```python
from build123d import *

# Parameters (mm, degrees)
F0_W     = 69.85
F0_H     = 95.25
F1_DEPTH = 38.1
F2_W     = 44.45
F2_H     = 73.66
F3_DEPTH = 25.4
F4_R     = 5.08
F5_R     = 4.826
F6_DEPTH = 12.7
F7_W     = 12.954
F7_H     = 6.35
F8_DEPTH = 12.7


# Not quite as in the source:
# - a feature names something its author has since deleted; it is built from what else it names


with BuildPart() as f1:
    # F0 (on Front) → F1 (new body)
    with BuildSketch(Plane.XZ):
        Rectangle(F0_W, F0_H)
    extrude(amount=F1_DEPTH)

    # F2 (on face) → F3 (cut)
    with BuildSketch(Plane(origin=(0, 0, 0), x_dir=(-1, 0, 0), z_dir=(0, 1, 0))):
        Rectangle(F2_W, F2_H)
    extrude(amount=-F3_DEPTH, mode=Mode.SUBTRACT)

    # F4
    f4_edges = [f1.edges().sort_by_distance(p)[0] for p in [
        (0, -38.1, 47.625),
        (0, 0, 47.625),
        (0, -38.1, -47.625),
        (0, 0, -47.625),
    ]]
    fillet(f4_edges, radius=F4_R)

    # F5 (on face) → F6 (cut)
    with BuildSketch(Plane.XZ.offset(38.1)):
        with Locations((-10.6567444081, 13.887990205)):
            Circle(F5_R)
        with Locations((9.5055226038, 14.3169752002)):
            Circle(F5_R)
    extrude(amount=-F6_DEPTH, mode=Mode.SUBTRACT)

    # F7 (on face) → F8 (cut)
    with BuildSketch(Plane.XZ.offset(38.1)):
        with Locations((0, -17.7338177471)):
            Rectangle(F7_W, F7_H)
    extrude(amount=-F8_DEPTH, mode=Mode.SUBTRACT)


solid = f1.part
```
Can you work these out from the model? Positions are in its coordinate system, mm. A direction names the side the tool comes from. Give positions to 0.01 mm unless a question says otherwise; leave off trailing zeros. Write each loop counter-clockwise with the first axis right and the second up, starting at its lowest first coordinate (ties: lowest second). Pieces come first, ordered by that corner, then holes. Notation, with made-up numbers: (-26.75, 24) -> (11.25, 24) arc R22 ccw to (11.25, 35) -> close; hole circle Ø10 at (-11, 24.5). An arc over 180 degrees is marked (long way). One line per item, written item: value.
Q1. Imagine slicing it at D-D on y = -31. Please give me the cut outline in (x, z) (3 decimals), and give its area (3 significant figures).
Results found:
outline: (-34.925, -47.625) -> (34.925, -47.625) -> (34.925, 47.625) -> (-34.925, 47.625) -> close; hole circle Ø9.652 at (-10.657, 13.888); hole (-6.477, -20.909) -> (6.477, -20.909) -> (6.477, -14.559) -> (-6.477, -14.559) -> close; hole circle Ø9.652 at (9.506, 14.317)
area: 6,420 mm^2
Q2. Imagine slicing it at A-A on x = -1.5. Please give me the cut outline in (y, z) (3 decimals).
Results found:
outline: (-38.1, -42.545) arc R5.08 ccw to (-33.02, -47.625) -> (-5.08, -47.625) arc R5.08 ccw to (0, -42.545) -> (0, -36.83) -> (-25.4, -36.83) -> (-25.4, -20.909) -> (-38.1, -20.909) -> close; (-38.1, -14.559) -> (-25.4, -14.559) -> (-25.4, 36.83) -> (0, 36.83) -> (0, 42.545) arc R5.08 ccw to (-5.08, 47.625) -> (-33.02, 47.625) arc R5.08 ccw to (-38.1, 42.545) -> close
Q3. For P1, Ø7.5, axis at x = 9.51, z = 14.32, coming from the +Y side, with a flat end and sliding along its axis, tell me the tip position at first contact or that it passes through.
Results found:
P1: passes through
Q4. Please list where these lines run through material, in increasing order: line 1 (X direction, y = -19, z = -2) (3 decimals); line 2 (Z direction, x = -12.5, y = -21.5) (3 decimals); line 3 (Y direction, x = -9, z = -1.5). Write a range as [from, to].
Results found:
line 1: x = [-34.925, -22.225], [22.225, 34.925]
line 2: z = [-47.625, -36.83], [36.83, 47.625]
line 3: y = [-38.1, -25.4]
Q5. We'd pull the mould along X, two halves only. Please class faces 4 (the face through (0, -38.1, 1)), 5 (the face through (0, -32, -20.909)), 6 (the face through (-34.925, -19, -1)), 7 (the face through (0, -13, 36.83)): +X half, -X half, draft (parallel to the pull), parting line (faces both ways), or undercut.
Results found:
face 4: draft
face 5: undercut
face 6: -X half
face 7: undercut
Q6. Imagine slicing it at B-B on z = -19. Please give me the cut outline in (x, y) (3 decimals).
Results found:
outline: (-34.925, -38.1) -> (-6.477, -38.1) -> (-6.477, -25.4) -> (-22.225, -25.4) -> (-22.225, 0) -> (-34.925, 0) -> close; (6.477, -38.1) -> (34.925, -38.1) -> (34.925, 0) -> (22.225, 0) -> (22.225, -25.4) -> (6.477, -25.4) -> close
Q7. Imagine slicing it at C-C on y = -20.5. Please give me the cut outline in (x, z) (3 decimals), and give its area (3 significant figures).
Results found:
outline: (-34.925, -47.625) -> (34.925, -47.625) -> (34.925, 47.625) -> (-34.925, 47.625) -> close; hole (-22.225, -36.83) -> (22.225, -36.83) -> (22.225, 36.83) -> (-22.225, 36.83) -> close
area: 3,380 mm^2
Q8. Which directions (+Z, -Z, +X, -X, +Y, -Y) give clear straight access to the entire face, cutting with the end or side of a thin tool? Please do faces 1 (the face through (0.49, -1.53, 46.18)), 2 (the face through (0, -32, -14.559)), 3 (the face through (22.225, -13, -1)).
Results found:
face 1: +Z, +X, -X, +Y
face 2: +Y, -Y
face 3: +Y
